CAD build for the part. Positions are in the model's coordinates, mm. Face numbers are marked on the shaded views. A direction names the side the tool comes from. Round coordinates to 2 decimals unless told otherwise and drop trailing zeros. Loops run counter-clockwise (first coordinate to the right, second up) from the corner with the lowest first, then second, coordinate; pieces in that order, holes last. Notation, with made-up numbers: M -39.75,-17 L -19.75,-17 A21 cw -19.75,-2 Z; hole C 16.25,-22 d11. An arc over 180 degrees is marked long. Use one line per item in the form item = value.
from build123d import *

# Parameters (mm, degrees)
SKETCH1_W           = 48.15
SKETCH1_H           = 26.17
BOSS_EXTRUDE1_DEPTH = 16.98
FILLET1_R           = 2
FILLET2_R           = 1
SKETCH2_R           = 3.665
SKETCH2_R_2         = 3.4
BOSS_EXTRUDE2_DEPTH = 3
FILLET6_R           = 0.3
FILLET10_R          = 0.1


with BuildPart() as part:
    # Sketch1 → Boss-Extrude1 (new body)
    with BuildSketch(Plane(origin=(0, 0, 0), x_dir=(1, 0, 0), z_dir=(0, 1, 0))):
        Rectangle(SKETCH1_W, SKETCH1_H)
    extrude(amount=BOSS_EXTRUDE1_DEPTH)

    # Fillet1
    fillet1_edges = [part.edges().sort_by_distance(p)[0] for p in [
        (0, 16.98, -13.085),
        (0, 0, -13.085),
        (0, 0, 13.085),
        (0, 16.98, 13.085),
    ]]
    fillet(fillet1_edges, radius=FILLET1_R)

    # Fillet2
    fillet2_edges = [part.edges().sort_by_distance(p)[0] for p in [
        (-24.075, 8.49, -13.085),
        (24.075, 8.49, -13.085),
        (-24.075, 0, 0),
        (-24.075, 8.49, 13.085),
        (-24.075, 16.98, 0),
        (-24.075, 16.394213562, 12.499213562),
        (-24.075, 16.394213562, -12.499213562),
        (-24.075, 0.585786438, 12.499213562),
        (-24.075, 0.585786438, -12.499213562),
        (24.075, 0, 0),
        (24.075, 16.98, 0),
        (24.075, 8.49, 13.085),
        (24.075, 16.394213562, 12.499213562),
        (24.075, 16.394213562, -12.499213562),
        (24.075, 0.585786438, 12.499213562),
        (24.075, 0.585786438, -12.499213562),
    ]]
    fillet(fillet2_edges, radius=FILLET2_R)

    # Sketch2 → Boss-Extrude2 (add)
    # profile 1 of 2: a face of its own
    with BuildSketch(Plane.ZY.offset(24.075)):
        with Locations(Location((-5.451156858, 8.49, 0), (0, 0, 180))):
            Circle(SKETCH2_R)
        with Locations((-5.451156858, 8.49)):
            Circle(SKETCH2_R_2, mode=Mode.SUBTRACT)
    # profile 2 of 2: a face of its own
    with BuildSketch(Plane.ZY.offset(24.075)):
        Polygon((4.510660825, 13.124360065), (0.610660825, 10.872694015), (0.610660825, 6.369361915), (4.510660825, 4.117695866), (8.410660825, 6.369361915), (8.410660825, 10.872694015), align=None)
        with Locations((4.510660825, 8.621027965)):
            Circle(SKETCH2_R, mode=Mode.SUBTRACT)
    extrude(amount=BOSS_EXTRUDE2_DEPTH)

    # Fillet6
    # the kernel refuses this fillet: 0.3 mm, written as the material it takes off along each edge
    with BuildSketch(Plane(origin=(-27.075, 8.621027965, 4.510660825), x_dir=(0, 0, 1), z_dir=(0, -1, 0))) as fillet6_piece_1:
        with BuildLine():
            CenterArc((3.665 + FILLET6_R, -FILLET6_R), FILLET6_R, 90, 90)
            Line((3.665, -FILLET6_R), (3.665, 0))
            Line((3.665, 0), (3.665 + FILLET6_R, 0))
        make_face()
    revolve(axis=Axis((-27.075, 8.621027965, 4.510660825), (-1, 0, 0)), mode=Mode.SUBTRACT)
    with BuildSketch(Plane(origin=(-27.075, 10.497694015, 9.060179878), x_dir=(1, 0, 0), z_dir=(0, 0.5000000000000002, -0.8660254037844386)), Plane(origin=(-27.075, 13.499360065, 5.160179878), x_dir=(1, 0, 0), z_dir=(0, -0.5000000000000002, -0.8660254037844386)), Plane(origin=(-27.075, 11.622694015, 0.610660825), x_dir=(1, 0, 0), z_dir=(0, -1, 0)), Plane(origin=(-27.075, 6.744361915, -0.038858228), x_dir=(1, 0, 0), z_dir=(0, -0.5000000000000002, 0.8660254037844386)), Plane(origin=(-27.075, 3.742695866, 3.861141772), x_dir=(1, 0, 0), z_dir=(0, 0.49999999999999983, 0.8660254037844388)), Plane(origin=(-27.075, 5.619361915, 8.410660825), x_dir=(1, 0, 0), z_dir=(0, 1, 0))) as fillet6_piece_2:
        with BuildLine():
            CenterArc((FILLET6_R, FILLET6_R), FILLET6_R, 180, 90)
            Line((0, FILLET6_R), (0, 0))
            Line((0, 0), (FILLET6_R, 0))
        make_face()
    extrude(amount=6.0033321, mode=Mode.SUBTRACT)

    # Fillet10
    fillet10_edges = [part.edges().sort_by_distance(p)[0] for p in [
        (-27.075, 8.49, -1.786156858),
        (-27.075, 8.49, -8.851156858),
    ]]
    fillet(fillet10_edges, radius=FILLET10_R)


solid = part.part
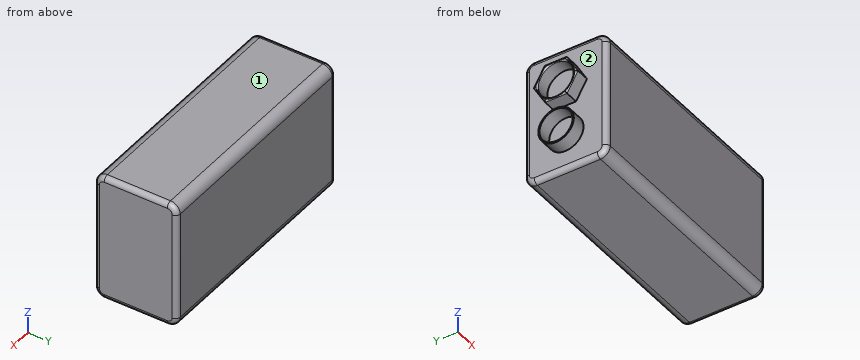
1. Cut at A-A on y = 2.75. Write the cut outline in (x, z) (3 decimals), and give its area (3 significant figures).
Completed:
outline = M -24.075,-12.085 A1 ccw -23.075,-13.085 L 23.075,-13.085 A1 ccw 24.075,-12.085 L 24.075,12.085 A1 ccw 23.075,13.085 L -23.075,13.085 A1 ccw -24.075,12.085 Z
area = 1,260 mm2
2. Drop flat-ended pins along their axis: P1, Ø2, axis at y = 9.5, z = 5.5, coming from the -X side (3 decimals); P2, Ø3, axis at x = -25, y = 9.5, coming from the -Z side. Give the stop position or say it passes through.
Completed:
P1 = -24.075
P2 = -12.99
3. Probe line 1 along X through (y, z) = (14, 10.5) (3 decimals); line 2 along Y through (x, z) = (-25, 2.75); line 3 along Z through (x, y) = (-6, 1.5). List the from-to ranges inside material, lowest first. Write a range as from..to.
Completed:
line_1 = -24.075..24.075
line_2 = 5.13..5.41, 11.84..12.11
line_3 = -13.02..13.02
4. Tool access for the marked faces 1 and 2: list every direction of +Z, -Z, +X, -X, +Y, -Y with a clear straight run to the whole face (end or side of a thin tool).
Completed:
face_1 = +Z, +X, -X, +Y, -Y
face_2 = -X
